```python
from build123d import *

# Parameters (mm, degrees)
SKETCH_2_R          = 100
SKETCH_2_R_2        = 3
SKETCH_2_R_3        = 30
EXTRUDE_1_DEPTH     = 20
SKETCH_3_R          = 43
CUT_EXTRUDE_1_DEPTH = 11
SKETCH_4_R          = 80
CUT_EXTRUDE_2_DEPTH = 6


with BuildPart() as part:
    # 草图2 → 凸台-拉伸1 (new body)
    with BuildSketch(Plane(origin=(0, 0, 0), x_dir=(1, 0, 0), z_dir=(0, 1, 0))):
        with Locations(Location((0, 0, 0), (0, 0, 270))):
            Circle(SKETCH_2_R)
        with Locations(Location((0, 90, 0), (0, 0, 270))):
            Circle(SKETCH_2_R_2, mode=Mode.SUBTRACT)
        with Locations(Location((90, 0, 0), (0, 0, 270))):
            Circle(SKETCH_2_R_2, mode=Mode.SUBTRACT)
        with Locations(Location((0, -90, 0), (0, 0, 270))):
            Circle(SKETCH_2_R_2, mode=Mode.SUBTRACT)
        with Locations(Location((-90, 0, 0), (0, 0, 270))):
            Circle(SKETCH_2_R_2, mode=Mode.SUBTRACT)
        with Locations(Location((0, 0, 0), (0, 0, 270))):
            Circle(SKETCH_2_R_3, mode=Mode.SUBTRACT)
    extrude(amount=EXTRUDE_1_DEPTH)

    # 草图3 → 切除-拉伸1 (cut)
    with BuildSketch(Plane.XZ):
        with Locations(Location((0, 0, 0), (0, 0, 270))):
            Circle(SKETCH_3_R)
    extrude(amount=-CUT_EXTRUDE_1_DEPTH, mode=Mode.SUBTRACT)

    # 草图4 → 切除-拉伸2 (cut)
    with BuildSketch(Plane(origin=(0, 20, 0), x_dir=(1, 0, 0), z_dir=(0, 1, 0))):
        with Locations(Location((0, 0, 0), (0, 0, 270))):
            Circle(SKETCH_4_R)
    extrude(amount=-CUT_EXTRUDE_2_DEPTH, mode=Mode.SUBTRACT)


solid = part.part
```
Geometry: final body of the model. Coordinates: model frame, mm. A direction names the side the tool comes from. Coordinates: 2 decimals unless noted, no trailing zeros. Loops run counter-clockwise (first coordinate to the right, second up) from the corner with the lowest first, then second, coordinate; pieces in that order, holes last. Notation, with made-up numbers: M 85.5,-22.5 L 107.5,-22.5 A4 cw 107.5,-18.5 Z; hole C -24.75,-11 d8. An arc over 180 degrees is marked long. Put each result on its own line as item: value.
(1) Cut plane A-A on x = 0. Return the cut outline in (y, z), then the cut area to 3 significant figures.
Answer sheet:
outline: M 0,-100 L 20,-100 L 20,-93 L 0,-93 Z; M 0,-87 L 20,-87 L 20,-80 L 14,-80 L 14,-30 L 11,-30 L 11,-43 L 0,-43 Z; M 0,43 L 11,43 L 11,30 L 14,30 L 14,80 L 20,80 L 20,87 L 0,87 Z; M 0,93 L 20,93 L 20,100 L 0,100 Z
area: 1,670 mm^2
(2) First-contact query: pin 1 (5 mm diameter, centred on x = -90, z = 0, fed in from +Y); pin 2 (8 mm diameter, centred on y = 4, z = -29.5, fed in from +X); pin 3 (6 mm diameter, centred on x = -40, y = 16.5, fed in from +Z); pin 4 (4 mm diameter, centred on x = -63.5, z = 15.5, fed in from +Y). Flat tips, straight axial feed; report the tip coordinate or a pass-through.
Answer sheet:
pin 1: passes through
pin 2: stops at x = 96.69
pin 3: stops at z = 92.9
pin 4: stops at y = 14
(3) Cut plane D-D on x = -24.5. Return the cut outline in (y, z), then the cut area to 3 significant figures.
Answer sheet:
outline: M 0,-96.95 L 20,-96.95 L 20,-76.16 L 14,-76.16 L 14,-17.31 L 11,-17.31 L 11,-35.34 L 0,-35.34 Z; M 0,35.34 L 11,35.34 L 11,17.31 L 14,17.31 L 14,76.16 L 20,76.16 L 20,96.95 L 0,96.95 Z
area: 2,080 mm^2
(4) Cut plane C-C on z = -16. Return the cut outline in (x, y), then the cut area to 3 significant figures.
Answer sheet:
outline: M -98.71,0 L -39.91,0 L -39.91,11 L -25.38,11 L -25.38,14 L -78.38,14 L -78.38,20 L -98.71,20 Z; M 25.38,11 L 39.91,11 L 39.91,0 L 98.71,0 L 98.71,20 L 78.38,20 L 78.38,14 L 25.38,14 Z
area: 1,980 mm^2
(5) Cut plane B-B on y = 3.75. Return the cut outline in (x, z), then the cut area to 3 significant figures.
Answer sheet:
outline: C 0,0 d200; hole C -90,0 d6; hole C 0,0 d86; hole C 0,-90 d6; hole C 0,90 d6; hole C 90,0 d6
area: 25,500 mm^2
(6) Material intervals for probe 1 along X at (y, z) = (16.7, 0); probe 2 along X at (y, z) = (13.15, 0); probe 3 along Y at (x, z) = (-19, 46), sorted ascending.
Answer sheet:
probe 1: x = -100 to -93, -87 to -80, 80 to 87, 93 to 100
probe 2: x = -100 to -93, -87 to -30, 30 to 87, 93 to 100
probe 3: y = 0 to 14
(7) Access query for faces 1 (the face through (-78.1, 17.04, -17.34)), 2 (the face through (29.061, 5.423, 31.693)), 3 (the face through (0, 10, 87)). Directions: +Z, -Z, +X, -X, +Y, -Y. A direction counts if a zero-diameter tool reaches every point of the face in a straight line with its end or side. Return the directions, or none.
Answer sheet:
face 1: +Y
face 2: -Y
face 3: +Y, -Y
(8) Draft query along Z for faces 4 (the face through (1.32, 12.48, -29.97)), 5 (the face through (75, 20, -30)), 6 (the face through (30.04, 9.86, 95.38)). Return one class per face: pulls with the +Z half, pulls with the -Z half, needs draft (parallel to the pull), parting line crosses it, or undercut.
Answer sheet:
face 4: undercut
face 5: needs draft
face 6: parting line crosses it
